```python
from build123d import *

# Parameters (mm, degrees)
BOSS_EXTRUDE1_DEPTH     = 3.81
TAP_DRILL_FOR_M3_TAP1_D = 2.5
F_3_0MM_DOWEL_HOLE1_D   = 3


with BuildPart() as part:
    # Sketch1 → Boss-Extrude1 (new body)
    with BuildSketch(Plane(origin=(0, 0, 0), x_dir=(0, 0, -1), z_dir=(1, 0, 0))):
        with BuildLine():
            Line((0, 0), (5.08, 0))
            ThreePointArc((5.08, 0), (11.43, 6.35), (5.08, 12.7))
            Line((5.08, 12.7), (0, 12.7))
            ThreePointArc((0, 12.7), (-6.35, 6.35), (0, 0))
        make_face()
    extrude(amount=BOSS_EXTRUDE1_DEPTH)

    # Tap Drill for M3 Tap1 (through all)
    with Locations(Plane(origin=(3.81, 0, 0), x_dir=(0, 0, -1), z_dir=(1, 0, 0))):
        with Locations((0, 6.35)):
            Hole(TAP_DRILL_FOR_M3_TAP1_D / 2)

    # Ø3.0mm Dowel Hole1 (through all)
    with Locations(Plane(origin=(3.81, 0, 0), x_dir=(0, 0, -1), z_dir=(1, 0, 0))):
        with Locations((5.08, 6.35)):
            Hole(F_3_0MM_DOWEL_HOLE1_D / 2)


solid = part.part
```
Design review of the part built by this model. Coordinates are the model's own, in mm. Round coordinates to 2 decimals unless told otherwise and drop trailing zeros. Order: outer loops, then holes, each group sorted by start corner. A loop starts at its lowest first (then second) coordinate and runs counter-clockwise, first axis right, second up. Notation, with made-up numbers: M 79,82 L 88,82 A26 cw 88,109 Z; hole C -1,-11.75 d5. An arc over 180 degrees is marked long. Put each result on its own line as item: value.
Q1. Consider section C-C (z = -4.5). State the section outline as (x, y) points.
Reported:
outline: M 0,0 L 3.81,0 L 3.81,4.97 L 0,4.97 Z; M 0,7.73 L 3.81,7.73 L 3.81,12.7 L 0,12.7 Z
Q2. Draft analysis for pull direction Y (two halves, no side actions). For faces 1 (the face through (1.88, 6.49, 6.35)), 2 (the face through (2, 12.7, -3)), 3 (the face through (1.88, 7.59, -0.16)), state which applies: released by +Y, released by -Y, zero draft, split by the parting line, or undercut.
Reported:
face 1: split by the parting line
face 2: released by +Y
face 3: undercut
Q3. Consider section D-D (z = -0.5). State the section outline as (x, y) points, and give its area (3 significant figures).
Reported:
outline: M 0,0 L 3.81,0 L 3.81,5.2 L 0,5.2 Z; M 0,7.5 L 3.81,7.5 L 3.81,12.7 L 0,12.7 Z
area: 39.7 mm²
Q4. Consider section A-A (y = 6.35). State the section outline as (x, z) points, and give its area (3 significant figures).
Reported:
outline: M 0,-11.43 L 3.81,-11.43 L 3.81,-6.58 L 0,-6.58 Z; M 0,-3.58 L 3.81,-3.58 L 3.81,-1.25 L 0,-1.25 Z; M 0,1.25 L 3.81,1.25 L 3.81,6.35 L 0,6.35 Z
area: 46.8 mm²
Q5. Insertion check: pin 1 Ø1 at (x, z) = (0.5, 2.5) entering from +Y. The pin has a flat end and moves straight along its axis. Give the tip position at first contact, or say it passes through.
Reported:
pin 1: y = 12.38
Q6. Consider section B-B (x = 0.8). State the section outline as (y, z) points, and give its area (3 significant figures).
Reported:
outline: M 0,-5.08 A6.35 ccw 12.7,-5.08 L 12.7,0 A6.35 ccw 0,0 Z; hole C 6.35,-5.08 d3; hole C 6.35,0 d2.5
area: 179 mm²
Q7. To check wall thickness, follow line 1 (Z direction, x = 1.85, y = 7.25); line 2 (Y direction, x = 2.3, z = -5.08); line 3 (Y direction, x = 3.65, z = -4.5). State the ranges of each line that lie inside material, in increasing order.
Reported:
line 1: -11.37 to -6.28, -3.88 to -0.87, 0.87 to 6.29
line 2: 0 to 4.85, 7.85 to 12.7
line 3: 0 to 4.97, 7.73 to 12.7
